Design review of the part shown in the three views and the two pictorial views. Dimensions are in mm from the part's minimum x, y and z. Round coordinates to 2 decimals unless told otherwise and drop trailing zeros. Order: outer loops, then holes, each group sorted by start corner. A loop starts at its lowest first (then second) coordinate and runs counter-clockwise, first axis right, second up.
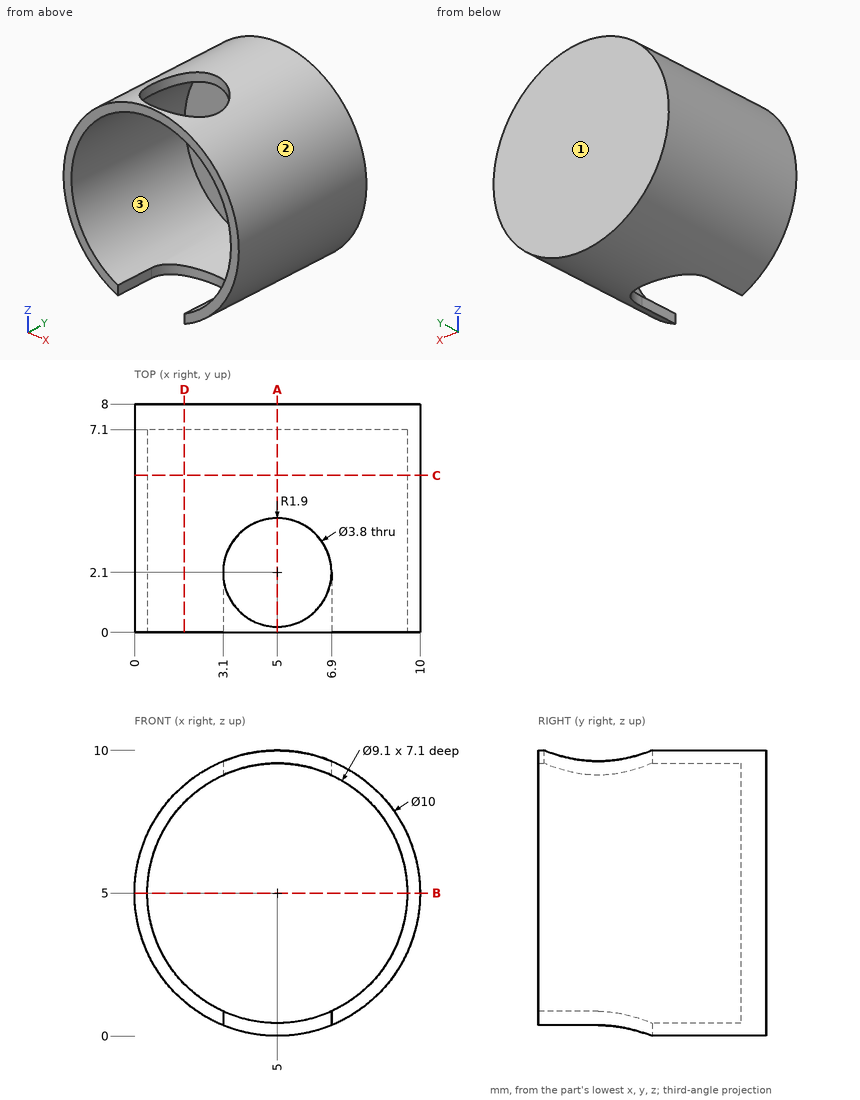
1) Take a section at B-B on z = 5. Give the boundary of the cut face in (x, y), plus the area to 3 significant figures.
Results:
outline: (0, 0) - (0.45, 0) - (0.45, 7.1) - (9.55, 7.1) - (9.55, 0) - (10, 0) - (10, 8) - (0, 8) - close
area: 15.4 mm2
2) To check wall thickness, follow line 1 along X through (y, z) = (4.5, 5); line 2 along Y through (x, z) = (2.5, 7); line 3 along X through (y, z) = (2.25, 2.25). State the ranges of each line that lie inside material, in increasing order.
Results:
line 1: x = 0 to 0.45, 9.55 to 10
line 2: y = 7.1 to 8
line 3: x = 0.82 to 1.38, 8.62 to 9.18
3) Clearance check with flat-ended pins moving along their axes: P1, Ø2, axis at y = 3.5, z = 8.5, coming from the -X side; P2, Ø2.5, axis at x = 5, y = 2.1, coming from the +Z side; P3, Ø3, axis at y = 5, z = 7.5, coming from the -X side; P4, Ø5, axis at x = 4.5, z = 6.5, coming from the -Y side. State where each tip first meets the part, or that it passes through.
Results:
P1: stops at x = 0.67
P2: passes through
P3: stops at x = 0.1
P4: stops at y = 7.1
4) Take a section at C-C on y = 5.5. Give the boundary of the cut face in (x, z), plus the area to 3 significant figures.
Results:
outline: circle Ø10 at (5, 5); hole circle Ø9.1 at (5, 5)
area: 13.5 mm2
5) The part is to be moulded in two halves that separate along X. For the marked faces 1, 2 and 3, say which applies: released by +X, released by -X, zero draft, split by the parting line, or undercut.
Results:
face 1: zero draft
face 2: split by the parting line
face 3: undercut
6) Take a section at D-D on x = 1.75. Give the boundary of the cut face in (y, z), plus the area to 3 significant figures.
Results:
outline: (0, 1.2) - (8, 1.2) - (8, 8.8) - (0, 8.8) - (0, 8.18) - (7.1, 8.18) - (7.1, 1.82) - (0, 1.82) - close
area: 15.6 mm2
7) Take a section at A-A on x = 5. Give the boundary of the cut face in (y, z).
Results:
outline: (0, 9.55) - (0.2, 9.55) - (0.2, 10) - (0, 10) - close; (4, 0) - (8, 0) - (8, 10) - (4, 10) - (4, 9.55) - (7.1, 9.55) - (7.1, 0.45) - (4, 0.45) - close
